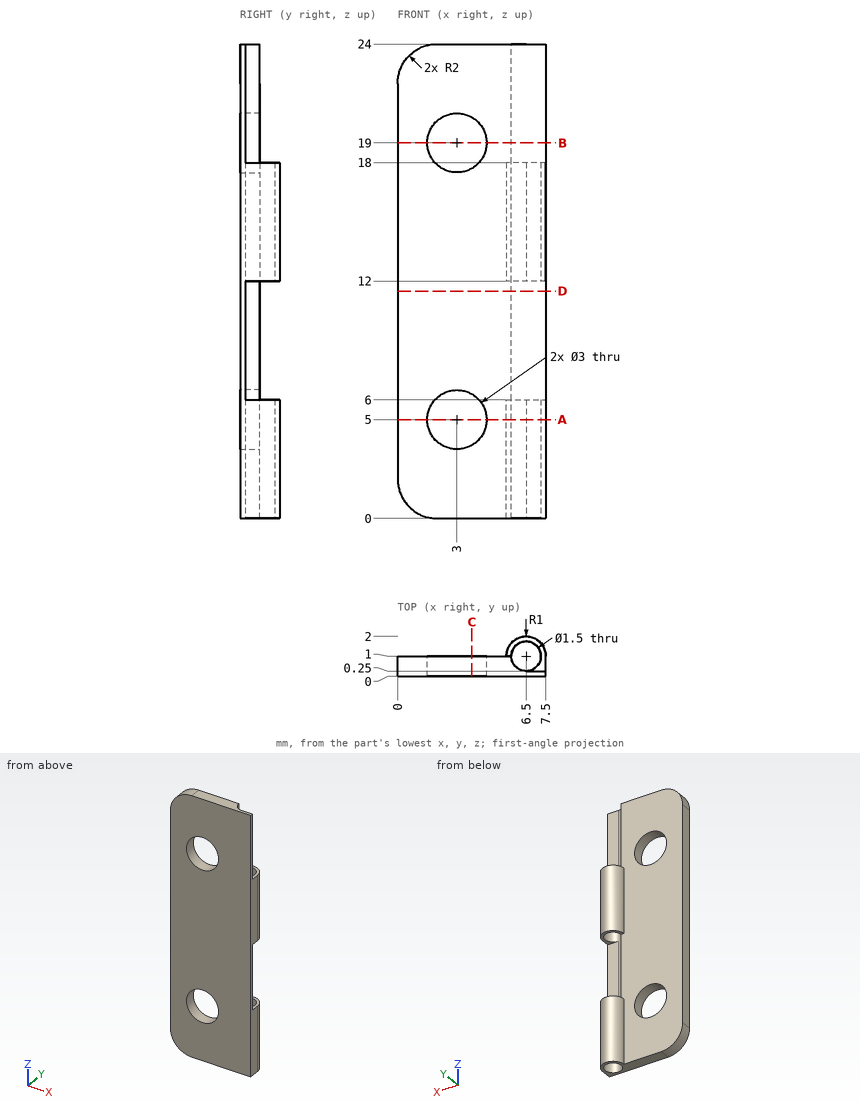
Geometry check sheet. Reference: drawing and pictorial views, mm from the part's lowest x, y, z. Round coordinates to 2 decimals unless told otherwise and drop trailing zeros. Loops run counter-clockwise (first coordinate to the right, second up) from the corner with the lowest first, then second, coordinate; pieces in that order, holes last. Notation, with made-up numbers: (60, 34) - (105, 34) arc R37 cw to (105, 73) - close; hole circle Ø2 at (51.25, 26.25). An arc over 180 degrees is marked (long way). Answer in a Markdown table with one row per item. Add a question column.
Q1. Section check D-D on z = 11.5. Enter the section's corners in (x, y).
Q2. Section check C-C on x = 3.75. Enter the section's corners in (y, z), plus the area to 3 significant figures.
Q3. Section check B-B on z = 19. Enter the section's corners in (x, y), plus the area to 3 significant figures.
Q4. Section check A-A on z = 5. Enter the section's corners in (x, y).
Q5. Gauge pin test, flat ends, axial feed: pin 1 (2 mm diameter, centred on x = 4.5, z = 21, fed in from +Y); pin 2 (1 mm diameter, centred on x = 1.5, y = 2, fed in from -Z); pin 3 (0.8 mm diameter, centred on x = 7, z = 22.5, fed in from +Y); pin 4 (0.9 mm diameter, centred on x = 7, y = 1.5, fed in from +Z). Record the tip position at first contact, or that the pin passes through.
Q6. Material ranges on line 1 (Z direction, x = 3.25, y = 0.4); line 2 (Y direction, x = 6.5, z = 12.5); line 3 (X direction, y = 0.85, z = 5), recorded low to high.
Found:
| question | item | result |
|---|---|---|
| 1 | outline | (0, 0) - (7.5, 0) - (7.5, 0.25) - (6.5, 0.25) arc R0.75 cw to (5.75, 1) - (0, 1) - close |
| 2 | outline | (0, 0) - (1, 0) - (1, 3.7) - (0, 3.7) - close; (0, 6.3) - (1, 6.3) - (1, 17.7) - (0, 17.7) - close; (0, 20.3) - (1, 20.3) - (1, 24) - (0, 24) - close |
| 2 | area | 18.8 mm² |
| 3 | outline | (0, 0) - (1.5, 0) - (1.5, 1) - (0, 1) - close; (4.5, 0) - (7.5, 0) - (7.5, 0.25) - (6.5, 0.25) arc R0.75 cw to (5.75, 1) - (4.5, 1) - close |
| 3 | area | 3.31 mm² |
| 4 | outline | (0, 0) - (1.5, 0) - (1.5, 1) - (0, 1) - close; (4.5, 0) - (7.5, 0) - (7.5, 1) arc R1 ccw to (5.5, 1) - (4.5, 1) - close; hole circle Ø1.5 at (6.5, 1) |
| 5 | pin 1 | stops at y = 1 |
| 5 | pin 2 | passes through |
| 5 | pin 3 | stops at y = 0.25 |
| 5 | pin 4 | stops at z = 18 |
| 6 | line 1 | z = 0 to 3.52, 6.48 to 17.52, 20.48 to 24 |
| 6 | line 2 | y = 0 to 0.25, 1.75 to 2 |
| 6 | line 3 | x = 0 to 1.5, 4.5 to 5.77, 7.23 to 7.5 |
